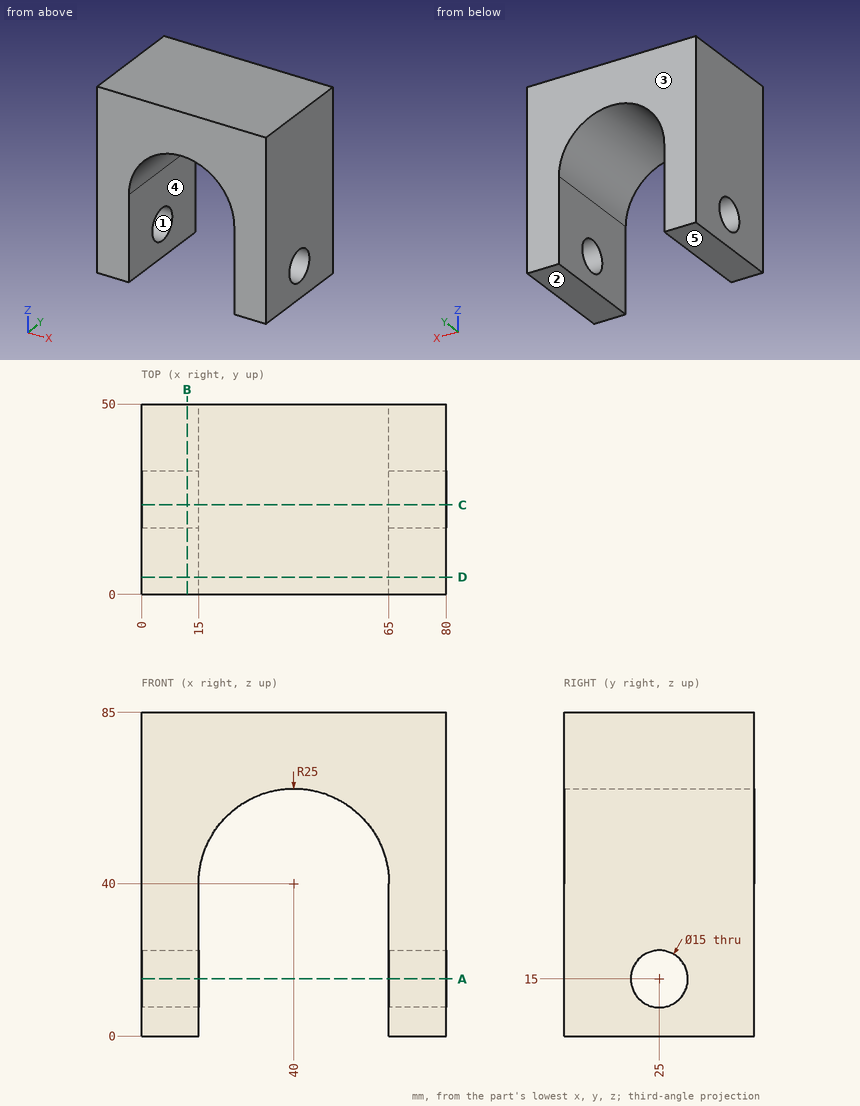
Verification items for this drawing (mm, ordinates from the low corner). A direction names the side the tool comes from. Give positions to 0.01 mm unless a question says otherwise; leave off trailing zeros. Order: outer loops, then holes, each group sorted by start corner. A loop starts at its lowest first (then second) coordinate and runs counter-clockwise, first axis right, second up.
1) Material ranges on probe 1 along X at (y, z) = (17, 33); probe 2 along Y at (x, z) = (74, 15); probe 3 along X at (y, z) = (40.5, 48), recorded low to high.
Results are:
probe 1: x = 0 to 15, 65 to 80
probe 2: y = 0 to 17.5, 32.5 to 50
probe 3: x = 0 to 16.31, 63.69 to 80
2) Cross-section at B-B (x = 12). Record the boundary of the cut face in (y, z), then the cut area to 3 significant figures.
Results are:
outline: (0, 0) - (50, 0) - (50, 85) - (0, 85) - close; hole circle Ø15 at (25, 15)
area: 4,070 mm2
3) Gauge pin test, flat ends, axial feed: pin 1 (4 mm diameter, centred on x = 63.5, z = 45, fed in from +Y); pin 2 (1.5 mm diameter, centred on x = 20, y = 44, fed in from -Z). Record the tip position at first contact, or that the pin passes through.
Results are:
pin 1: stops at y = 50
pin 2: stops at z = 53.94
4) Cross-section at C-C (y = 23.5). Record the boundary of the cut face in (x, z), then the cut area to 3 significant figures.
Results are:
outline: (0, 0) - (15, 0) - (15, 7.65) - (0, 7.65) - close; (0, 22.35) - (15, 22.35) - (15, 40) arc R25 cw to (65, 40) - (65, 22.35) - (80, 22.35) - (80, 85) - (0, 85) - close; (65, 0) - (80, 0) - (80, 7.65) - (65, 7.65) - close
area: 3,380 mm2
5) Tool access check on the marked faces 4 and 5. Record the directions out of +Z, -Z, +X, -X, +Y, -Y that give a thin tool (end or side, any length) a straight path to the whole face; none if there is none.
Results are:
face 4: -Z, +Y, -Y
face 5: -Z, +X, -X, +Y, -Y
6) Draft check along Y on the marked faces 1, 2 and 3. Enter one of: released by +Y, released by -Y, zero draft, split by the parting line, or undercut.
Results are:
face 1: undercut
face 2: zero draft
face 3: released by +Y
7) Cross-section at A-A (z = 15). Record the boundary of the cut face in (x, y).
Results are:
outline: (0, 0) - (15, 0) - (15, 17.5) - (0, 17.5) - close; (0, 32.5) - (15, 32.5) - (15, 50) - (0, 50) - close; (65, 0) - (80, 0) - (80, 17.5) - (65, 17.5) - close; (65, 32.5) - (80, 32.5) - (80, 50) - (65, 50) - close
8) Cross-section at D-D (y = 4.5). Record the boundary of the cut face in (x, z).
Results are:
outline: (0, 0) - (15, 0) - (15, 40) arc R25 cw to (65, 40) - (65, 0) - (80, 0) - (80, 85) - (0, 85) - close
